Part model, mm, in its own coordinate system. A direction names the side the tool comes from. Round coordinates to 2 decimals unless told otherwise and drop trailing zeros. Loops run counter-clockwise (first coordinate to the right, second up) from the corner with the lowest first, then second, coordinate; pieces in that order, holes last. Notation, with made-up numbers: (-26.5, 71) - (32.5, 71) arc R36 cw to (32.5, 109) - close; hole circle Ø2 at (85, -36). An arc over 180 degrees is marked (long way). Put each result on its own line as item: value.
from build123d import *

# Parameters (mm, degrees)
BOSS_EXTRUDE1_DEPTH = 3


with BuildPart() as part:
    # Sketch1 → Boss-Extrude1 (new body)
    with BuildSketch(Plane(origin=(0, 0, 0), x_dir=(1, 0, 0), z_dir=(0, 1, 0))):
        with BuildLine():
            Line((0, 0), (-40, 0))
            ThreePointArc((-40, 0), (-43, 3), (-40, 6))
            Line((-40, 6), (0, 6))
            ThreePointArc((0, 6), (3, 3), (0, 0))
        make_face()
        with BuildLine():
            Line((-40, 4.5), (-34, 4.5))
            ThreePointArc((-34, 4.5), (-32.5, 3), (-34, 1.5))
            Line((-34, 1.5), (-40, 1.5))
            ThreePointArc((-40, 1.5), (-41.5, 3), (-40, 4.5))
        make_face(mode=Mode.SUBTRACT)
        with BuildLine():
            Line((0, 1.5), (-6, 1.5))
            ThreePointArc((-6, 1.5), (-7.5, 3), (-6, 4.5))
            Line((-6, 4.5), (0, 4.5))
            ThreePointArc((0, 4.5), (1.5, 3), (0, 1.5))
        make_face(mode=Mode.SUBTRACT)
    extrude(amount=BOSS_EXTRUDE1_DEPTH)


solid = part.part
1. Band-saw the part on B-B (y = 1.1). List the corners of the cut face in (x, z).
A:
outline: (-40, -6) - (0, -6) arc R3 ccw to (0, 0) - (-40, 0) arc R3 ccw to start; hole (-40, -4.5) - (-34, -4.5) arc R1.5 ccw to (-34, -1.5) - (-40, -1.5) arc R1.5 ccw to start; hole (-6, -4.5) - (0, -4.5) arc R1.5 ccw to (0, -1.5) - (-6, -1.5) arc R1.5 ccw to start
2. Band-saw the part on A-A (x = -5). List the corners of the cut face in (y, z).
A:
outline: (0, -6) - (3, -6) - (3, -4.5) - (0, -4.5) - close; (0, -1.5) - (3, -1.5) - (3, 0) - (0, 0) - close
3. Band-saw the part on C-C (z = -2). List the corners of the cut face in (x, y), plus the area to 3 significant figures.
A:
outline: (-42.83, 0) - (-41.12, 0) - (-41.12, 3) - (-42.83, 3) - close; (-32.88, 0) - (-7.12, 0) - (-7.12, 3) - (-32.88, 3) - close; (1.12, 0) - (2.83, 0) - (2.83, 3) - (1.12, 3) - close
area: 87.6 mm²
4. Band-saw the part on D-D (z = -5.1). List the corners of the cut face in (x, y), plus the area to 3 significant figures.
A:
outline: (-42.14, 0) - (2.14, 0) - (2.14, 3) - (-42.14, 3) - close
area: 133 mm²
5. Tool access for faces 1 (the flat face through (-37, 1, -4.5)), 2 (the flat face through (-20, 0, -3)): list every direction of +Z, -Z, +X, -X, +Y, -Y with a clear straight run to the whole face (end or side of a thin tool).
A:
face 1: +Y, -Y
face 2: +Z, -Z, +X, -X, -Y
6. Two-plate mould, pull along Z, no slides. Class faces 3 (the flat face through (-20, 1, 0)), 4 (the cylindrical face through (3, 1, -3)), 5 (the flat face through (-3, 1, -4.5)): pulls with the +Z half, pulls with the -Z half, needs draft (parallel to the pull), parting line crosses it, or undercut.
A:
face 3: pulls with the +Z half
face 4: parting line crosses it
face 5: undercut
7. Pin check, flat tip, straight feed: P1, Ø1.5, axis at y = 1, z = -5, coming from the -X side. Stop position of the tip, or through.
A:
P1: stops at x = -42.73
8. Probe line 1 along X through (y, z) = (1.55, -3); line 2 along Z through (x, y) = (-5, 1.1); line 3 along X through (y, z) = (1.45, -2.1). List the from-to ranges inside material, lowest first. Write a range as [from, to].
A:
line 1: x = [-43, -41.5], [-32.5, -7.5], [1.5, 3]
line 2: z = [-6, -4.5], [-1.5, 0]
line 3: x = [-42.86, -41.2], [-32.8, -7.2], [1.2, 2.86]
